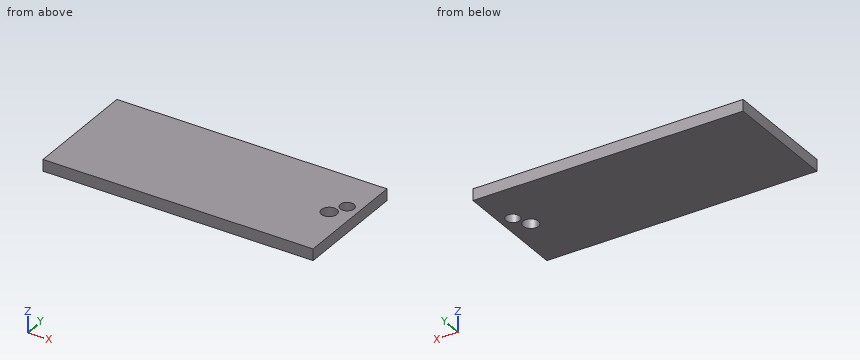
```python
from build123d import *

# Parameters (mm, degrees)
ESQUISSE1_W             = 350
ESQUISSE1_H             = 150
BOSS_EXTRU_1_DEPTH      = 15
ESQUISSE2_R             = 10
ENL_V_MAT_EXTRU_2_DEPTH = 382.083980246
ESQUISSE3_R             = 9
ENL_V_MAT_EXTRU_3_DEPTH = 20


with BuildPart() as part:
    # Esquisse1 → Boss.-Extru.1 (new body)
    with BuildSketch(Plane.XY):
        with Locations((175, -75)):
            Rectangle(ESQUISSE1_W, ESQUISSE1_H)
    extrude(amount=BOSS_EXTRU_1_DEPTH)

    # Esquisse2 → Enlèv. mat.-Extru.2 (cut, through all)
    with BuildSketch(Plane(origin=(0, 0, 0), x_dir=(-1, 0, 0), z_dir=(0, 0, -1))):
        with Locations((-323, -75)):
            Circle(ESQUISSE2_R)
    extrude(amount=-ENL_V_MAT_EXTRU_2_DEPTH, mode=Mode.SUBTRACT)

    # Esquisse3 → Enlèv. mat.-Extru.3 (cut)
    with BuildSketch(Plane.XY.offset(15)):
        with Locations((333.5, -54.976135627)):
            Circle(ESQUISSE3_R)
    extrude(amount=-ENL_V_MAT_EXTRU_3_DEPTH, mode=Mode.SUBTRACT)


solid = part.part
```
Geometry: final body of the model. Coordinates: model frame, mm. Coordinates: 2 decimals unless noted, no trailing zeros. Order: outer loops, then holes, each group sorted by start corner. A loop starts at its lowest first (then second) coordinate and runs counter-clockwise, first axis right, second up. Notation, with made-up numbers: (7.25, 49) - (29.25, 49) arc R25 ccw to (29.25, 84) - close; hole circle Ø3 at (-30, 7). An arc over 180 degrees is marked (long way). Return JSON: item names as keys, results as strings. Group by question number.
1. Material intervals for line 1 along Y through (x, z) = (333.5, 7); line 2 along Y through (x, z) = (323, 11.5); line 3 along X through (y, z) = (-60.5, 10.25), sorted ascending. Write a range as [from, to].
2. Cut plane A-A (y = -75). Output: boundary loops of the cut face in (x, z), plus the area to 3 significant figures.
3. Pin query (flat end, axial travel): pin 1 (16 mm diameter, centred on x = 333.5, y = -54.98, fed in from +Z). Return the tip coordinate at first contact, or that it passes through.
4. Cut plane B-B (x = 328.5). Output: boundary loops of the cut face in (y, z).
Resolved:
{
 "1": {"line 1": "y = [-150, -63.98], [-45.98, 0]", "line 2": "y = [-150, -85], [-65, 0]", "line 3": "x = [0, 326.39], [340.61, 350]"},
 "2": {"outline": "(0, 0) - (313, 0) - (313, 15) - (0, 15) - close; (333, 0) - (350, 0) - (350, 15) - (333, 15) - close", "area": "4,950 mm²"},
 "3": {"pin 1": "passes through"},
 "4": {"outline": "(-150, 0) - (-83.35, 0) - (-83.35, 15) - (-150, 15) - close; (-66.65, 0) - (-62.46, 0) - (-62.46, 15) - (-66.65, 15) - close; (-47.49, 0) - (0, 0) - (0, 15) - (-47.49, 15) - close"}
}
